Geometry check sheet. Reference: drawing and pictorial views, mm from the part's lowest x, y, z. A direction names the side the tool comes from. Coordinates: 2 decimals unless noted, no trailing zeros. Loops run counter-clockwise (first coordinate to the right, second up) from the corner with the lowest first, then second, coordinate; pieces in that order, holes last. Notation, with made-up numbers: (82.25, 77.25) - (94.25, 77.25) arc R13 cw to (94.25, 84.25) - close; hole circle Ø8 at (15, 11.5). An arc over 180 degrees is marked (long way). One line per item, written item: value.
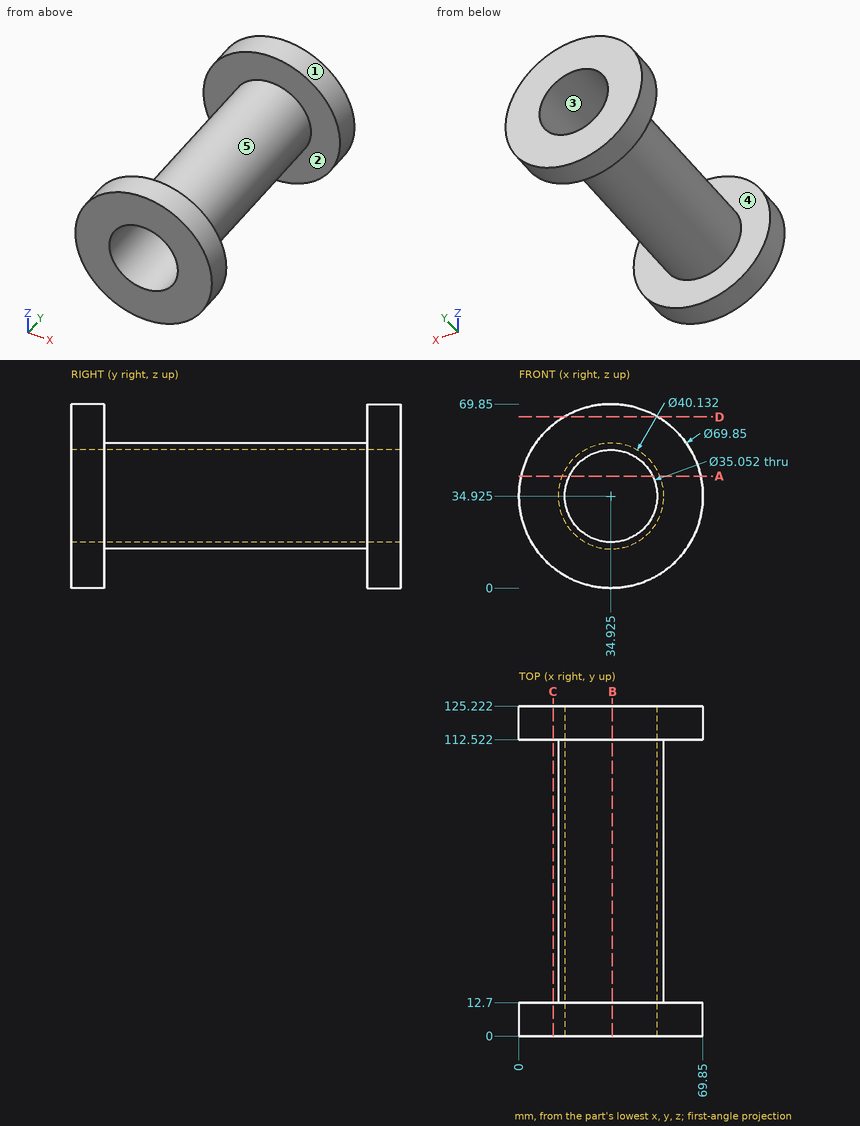
(1) Material ranges on probe 1 along Y at (x, z) = (63, 44.5); probe 2 along X at (y, z) = (27.5, 45); probe 3 along Z at (x, y) = (19, 62), recorded low to high. Write a range as from..to.
Reply:
probe 1: 0..12.7, 112.52..125.22
probe 2: 17.57..20.58, 49.27..52.28
probe 3: 22.72..27.61, 42.24..47.13
(2) Go/stop test with flat-tipped pins: pin 1 Ø6 at (y, z) = (87.5, 54.5) entering from -X; pin 2 Ø12 at (y, z) = (45, 32) entering from +X; pin 3 Ø5 at (y, z) = (97.5, 22) entering from +X. Record where each tip stops, or that it passes through.
Reply:
pin 1: x = 23.62
pin 2: x = 54.99
pin 3: x = 52.07
(3) Release check for a two-part mould opening along X. For the marked faces 3, 4 and 5 record: pulls with the +X half, pulls with the -X half, needs draft (parallel to the pull), parting line crosses it, or undercut.
Reply:
face 3: undercut
face 4: needs draft
face 5: parting line crosses it
(4) Cross-section at D-D on z = 65. Record the cut outline in (x, y).
Reply:
outline: (17.17, 0) - (52.68, 0) - (52.68, 12.7) - (17.17, 12.7) - close; (17.17, 112.52) - (52.68, 112.52) - (52.68, 125.22) - (17.17, 125.22) - close
(5) Cross-section at C-C on x = 13. Record the cut outline in (y, z), and give its area (3 significant figures).
Reply:
outline: (0, 7.74) - (12.7, 7.74) - (12.7, 62.11) - (0, 62.11) - close; (112.52, 7.74) - (125.22, 7.74) - (125.22, 62.11) - (112.52, 62.11) - close
area: 1,380 mm2
(6) Cross-section at B-B on x = 35.5. Record the cut outline in (y, z), and give its area (3 significant figures).
Reply:
outline: (0, 0) - (12.7, 0) - (12.7, 14.87) - (112.52, 14.87) - (112.52, 0) - (125.22, 0) - (125.22, 17.41) - (0, 17.41) - close; (0, 52.44) - (125.22, 52.44) - (125.22, 69.85) - (112.52, 69.85) - (112.52, 54.98) - (12.7, 54.98) - (12.7, 69.85) - (0, 69.85) - close
area: 1,390 mm2
(7) Access from +Z, -Z, +X, -X, +Y, -Y to the whole of each face (thin tool, end or side, straight path). Record for the marked faces 1 and 2.
Reply:
face 1: +Y, -Y
face 2: none
(8) Cross-section at A-A on z = 42.5. Record the cut outline in (x, y).
Reply:
outline: (0.83, 0) - (19.12, 0) - (19.12, 125.22) - (0.83, 125.22) - (0.83, 112.52) - (16.34, 112.52) - (16.34, 12.7) - (0.83, 12.7) - close; (50.73, 0) - (69.02, 0) - (69.02, 12.7) - (53.51, 12.7) - (53.51, 112.52) - (69.02, 112.52) - (69.02, 125.22) - (50.73, 125.22) - close
